from build123d import *

# Parameters (mm, degrees)
EXTRUDE_1_DEPTH     = 5
SKETCH_2_5_R        = 0.5
CUT_EXTRUDE_1_DEPTH = 6
EXTRUDE_2_DEPTH     = 4
SKETCH_2_8_R        = 2
CUT_EXTRUDE_2_DEPTH = 4
SKETCH_3_R          = 3.5
EXTRUDE_3_DEPTH     = 15
EXTRUDE_4_DEPTH     = 22
SKETCH_5_R          = 3
EXTRUDE_5_DEPTH     = 16
EXTRUDE_5_TAPER     = 4
SKETCH_6_R          = 3
EXTRUDE_6_DEPTH     = 16
EXTRUDE_6_TAPER     = 4
SKETCH_7_R          = 4.663684065
EXTRUDE_7_DEPTH     = 16


with BuildPart() as part:
    # 草图2 → 凸台-拉伸1 (new body)
    with BuildSketch(Plane.XY):
        with BuildLine():
            Line((15.641000066, 15.243423767), (15.641000066, 3.009489297))
            ThreePointArc((15.641000066, 3.009489297), (16.763817885, 0.66936386), (19.291791439, 0.080928117))
            Line((19.291791439, 0.080928117), (22.370518946, 0.765089785))
            ThreePointArc((22.370518946, 0.765089785), (24.059853009, 1.816468785), (24.719727573, 3.693650965))
            Line((24.719727573, 3.693650965), (24.719727573, 14.880621327))
            ThreePointArc((24.719727573, 14.880621327), (24.059853009, 16.757803508), (22.370518946, 17.809182508))
            Line((22.370518946, 17.809182508), (19.605498159, 18.423631571))
            ThreePointArc((19.605498159, 18.423631571), (16.860299842, 17.784632476), (15.641000066, 15.243423767))
        make_face()
    extrude(amount=EXTRUDE_1_DEPTH)

    # 草图2<5> → 切除-拉伸1 (cut)
    with BuildSketch(Plane.XY):
        with Locations((18.898785314, 15.243423767)):
            Circle(SKETCH_2_5_R)
        with Locations((18.898785314, 12.243423767)):
            Circle(SKETCH_2_5_R)
        with Locations((18.898785314, 9.096563263)):
            Circle(SKETCH_2_5_R)
        with Locations((18.898785314, 6.048083228)):
            Circle(SKETCH_2_5_R)
        with Locations((18.898785314, 3.009489297)):
            Circle(SKETCH_2_5_R)
        with Locations((21.228436708, 13.929259558)):
            Circle(SKETCH_2_5_R)
        with Locations((21.228436708, 10.621115871)):
            Circle(SKETCH_2_5_R)
        with Locations((21.228436708, 7.588650825)):
            Circle(SKETCH_2_5_R)
        with Locations((21.228436708, 4.494923859)):
            Circle(SKETCH_2_5_R)
    extrude(amount=CUT_EXTRUDE_1_DEPTH, mode=Mode.SUBTRACT)

    # 草图2<6> → 凸台-拉伸2 (add)
    with BuildSketch(Plane.XY):
        Polygon((12.719727573, 9.287136146), (12.719727573, 25.787136146), (26.719727573, 25.787136146), (26.719727573, -7.212863854), (12.719727573, -7.212863854), align=None)
    extrude(amount=-EXTRUDE_2_DEPTH)

    # 草图2<8> → 切除-拉伸2 (cut)
    with BuildSketch(Plane.XY):
        with Locations((19.719727573, -3.681329619)):
            Circle(SKETCH_2_8_R)
        with Locations((19.719727573, 22.255849174)):
            Circle(SKETCH_2_8_R)
    extrude(amount=-CUT_EXTRUDE_2_DEPTH, mode=Mode.SUBTRACT)

    # 草图3 → 凸台-拉伸3 (add)
    with BuildSketch(Plane(origin=(0, 0, -4), x_dir=(-1, 0, 0), z_dir=(0, 0, -1))):
        with Locations((-19.719727573, 22.255849174)):
            Circle(SKETCH_3_R)
        with Locations((-19.719727573, -3.681329619)):
            Circle(SKETCH_3_R)
    extrude(amount=EXTRUDE_3_DEPTH)

    # 草图4 → 凸台-拉伸4 (add)
    with BuildSketch(Plane(origin=(0, 0, -4), x_dir=(-1, 0, 0), z_dir=(0, 0, -1))):
        with BuildLine():
            Line((-23.719727573, 19.091579688), (-15.719727573, 19.091579688))
            ThreePointArc((-15.719727573, 19.091579688), (-13.598407229, 18.212900031), (-12.719727573, 16.091579688))
            Line((-12.719727573, 16.091579688), (-12.719727573, 2.402820502))
            ThreePointArc((-12.719727573, 2.402820502), (-13.598407229, 0.281500159), (-15.719727573, -0.597179498))
            Line((-15.719727573, -0.597179498), (-23.719727573, -0.597179498))
            ThreePointArc((-23.719727573, -0.597179498), (-25.841047916, 0.281500159), (-26.719727573, 2.402820502))
            Line((-26.719727573, 2.402820502), (-26.719727573, 16.091579688))
            ThreePointArc((-26.719727573, 16.091579688), (-25.841047916, 18.212900031), (-23.719727573, 19.091579688))
        make_face()
    extrude(amount=EXTRUDE_4_DEPTH)

    # 草图5 → 凸台-拉伸5 (add)
    with BuildSketch(Plane(origin=(0, 0, -19), x_dir=(-1, 0, 0), z_dir=(0, 0, -1))):
        with Locations((-19.719727573, 22.255849174)):
            Circle(SKETCH_5_R)
    extrude(amount=EXTRUDE_5_DEPTH, taper=EXTRUDE_5_TAPER)

    # 草图6 → 凸台-拉伸6 (add)
    with BuildSketch(Plane(origin=(0, 0, -19), x_dir=(-1, 0, 0), z_dir=(0, 0, -1))):
        with Locations((-19.719727573, -3.681329619)):
            Circle(SKETCH_6_R)
    extrude(amount=EXTRUDE_6_DEPTH, taper=EXTRUDE_6_TAPER)

    # 草图7 → 凸台-拉伸7 (add)
    with BuildSketch(Plane(origin=(0, 0, -26), x_dir=(-1, 0, 0), z_dir=(0, 0, -1))):
        with Locations((-19.855274078, 10.100415179)):
            Circle(SKETCH_7_R)
    extrude(amount=EXTRUDE_7_DEPTH)


solid = part.part
CAD build for the part. Positions are in the model's coordinates, mm. A direction names the side the tool comes from. Give positions to 0.01 mm unless a question says otherwise; leave off trailing zeros. Write each loop counter-clockwise with the first axis right and the second up, starting at its lowest first coordinate (ties: lowest second). Pieces come first, ordered by that corner, then holes. Notation, with made-up numbers: M -22.5,86 L -15.5,86 A28 ccw -15.5,110 Z; hole C 40.5,43 d10. An arc over 180 degrees is marked long. Put each result on its own line as item: value. Start each with the question number.
(1) Probe L1, parallel to Y at x = 21.5, z = 1.5; L2, parallel to Y at x = 20.5, z = -22.5; L3, parallel to Y at x = 22.25, z = -8.5. List the from-to ranges inside material, lowest first.
(2) Flat gauge pins, fed straight in: pin 1 Ø1.2 at (x, y) = (20, -3) entering from +Z; pin 2 Ø5.5 at (x, y) = (19.5, 21) entering from -Z; pin 3 Ø3 at (y, z) = (6, -36) entering from +X; pin 4 Ø2 at (y, z) = (0.5, -29.5) entering from -X. Where does each tip first touch, or does it go through?
(3) Band-saw the part on B-B, the plane x = 14.25. Write the cut outline in (y, z).
(4) Band-saw the part on A-A, the plane z = -20. Write the cut outline in (x, y).
(5) Band-saw the part on D-D, the plane z = -39. Write the cut outline in (x, y), and give its area (3 significant figures).
(6) Band-saw the part on C-C, the plane z = -2.5. Write the cut outline in (x, y).
(7) Which spindle directions (+Z, -Z, +X, -X, +Y, -Y) get a long thin tool onto all of the face, cutting with end or side? Do faces 1 (the face through (24.72, 9, 2)), 2 (the face through (13.622, 18.236, -14.846)), 3 (the face through (17.3, 14, -33.9)), 4 (the face through (19, 9, 0)), 5 (the face through (20.81, 0.42, 2.46)). Say none if no direction does.
Response values:
1. L1: y = 0.57 to 4.08, 4.91 to 7.17, 8.01 to 10.2, 11.04 to 13.51, 14.35 to 18
1. L2: y = -6.32 to -1.04, -0.6 to 19.09, 19.61 to 24.9
1. L3: y = -6.1 to -1.26, -0.6 to 19.09, 19.84 to 24.67
2. pin 1: stops at z = -4
2. pin 2: stops at z = -35
2. pin 3: stops at x = 23.73
2. pin 4: passes through
3. outline: M -7.21,-4 L -0.21,-4 L -0.21,-26 L 18.71,-26 L 18.71,-4 L 25.79,-4 L 25.79,0 L -7.21,0 Z
4. outline: M 12.72,2.4 A3 ccw 15.72,-0.6 L 23.72,-0.6 A3 ccw 26.72,2.4 L 26.72,16.09 A3 ccw 23.72,19.09 L 15.72,19.09 A3 ccw 12.72,16.09 Z; C 19.72,-3.68 d5.86; C 19.72,22.26 d5.86
5. outline: C 19.86,10.1 d9.33
5. area: 68.3 mm2
6. outline: M 12.72,-7.21 L 26.72,-7.21 L 26.72,25.79 L 12.72,25.79 Z; hole C 19.72,-3.68 d4; hole C 19.72,22.26 d4
7. face 1: +Z, +X, +Y, -Y
7. face 2: -Z, -X, +Y
7. face 3: -Z
7. face 4: +Z
7. face 5: +Z, +X, -Y
